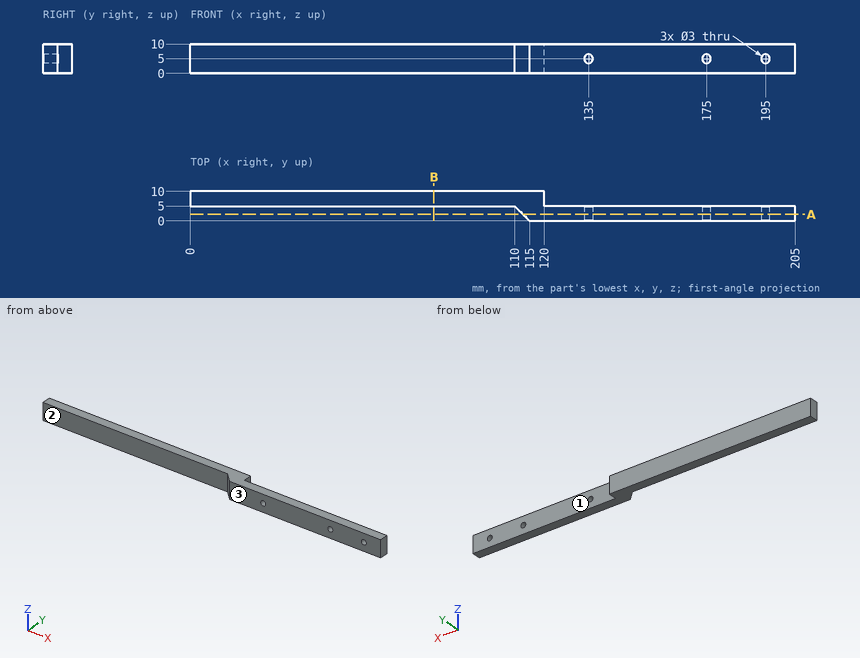
Check sheet for the drawn part. Datum: minimum x, y, z corner. Units: mm. A direction names the side the tool comes from. Round coordinates to 2 decimals unless told otherwise and drop trailing zeros. Order: outer loops, then holes, each group sorted by start corner. A loop starts at its lowest first (then second) coordinate and runs counter-clockwise, first axis right, second up. Notation, with made-up numbers: (77.5, 88.5) -> (133.5, 88.5) arc R13 ccw to (133.5, 92.5) -> close; hole circle Ø5 at (82, 62). An arc over 180 degrees is marked (long way). Put each result on its own line as item: value. Start each with the question number.
(1) Depth check by flat-ended pin: pin 1 Ø3 at (x, z) = (173, 4) entering from +Y; pin 2 Ø6 at (x, z) = (79, 8.5) entering from -Y. Enter the tip coordinate at first touch or a pass-through.
(2) Section check A-A (y = 2.25). Enter the section's corners in (x, z), then the cut area to 3 significant figures.
(3) Tool access check on the marked faces 1, 2 and 3. Record the directions out of +Z, -Z, +X, -X, +Y, -Y that give a thin tool (end or side, any length) a straight path to the whole face; none if there is none.
(4) Section check B-B (x = 82.5). Enter the section's corners in (y, z).
(5) Material ranges on line 1 along Z through (x, y) = (135, 3.7); line 2 along X through (y, z) = (1.75, 3.75); line 3 along X through (y, z) = (7.75, 6.5), recorded low to high.
Completed:
1. pin 1: stops at y = 5
1. pin 2: stops at y = 5
2. outline: (112.75, 0) -> (205, 0) -> (205, 10) -> (112.75, 10) -> close; hole circle Ø3 at (135, 5); hole circle Ø3 at (175, 5); hole circle Ø3 at (195, 5)
2. area: 901 mm2
3. face 1: +Z, -Z, +X, +Y
3. face 2: +Z, -Z, -X, -Y
3. face 3: +Z, -Z, +X, -X, -Y
4. outline: (5, 0) -> (10, 0) -> (10, 10) -> (5, 10) -> close
5. line 1: z = 0 to 3.5, 6.5 to 10
5. line 2: x = 113.25 to 134.17, 135.83 to 174.17, 175.83 to 194.17, 195.83 to 205
5. line 3: x = 0 to 120
